Here's how the part is built. I have some questions about the finished solid (model axes, mm). A direction names the side the tool comes from. Give positions to 0.01 mm unless a question says otherwise; leave off trailing zeros. Order: outer loops, then holes, each group sorted by start corner. A loop starts at its lowest first (then second) coordinate and runs counter-clockwise, first axis right, second up.
from build123d import *

# Parameters (mm, degrees)
F0_R     = 25.4
F1_DEPTH = 142.875
F2_R     = 5.5626
F3_DEPTH = 6.35
F4_R     = 2.413
F5_DEPTH = 9.525


with BuildPart() as f1:
    # F0 (on Top) → F1 (new body)
    with BuildSketch(Plane.XY):
        Circle(F0_R)
    extrude(amount=F1_DEPTH)

    # F2 (on face) → F3 (join)
    with BuildSketch(Plane.XY.offset(142.875)):
        with Locations((-11.1125, 0)):
            Circle(F2_R)
    extrude(amount=F3_DEPTH)

    # F4 (on face) → F5 (cut)
    with BuildSketch(Plane.XY.offset(149.225)):
        with Locations((-11.1125, 0)):
            Circle(F4_R)
    extrude(amount=-F5_DEPTH, mode=Mode.SUBTRACT)

    # F6: F1 across plane


with BuildPart() as f1_1:
    add(f1.part)
    add(f1.part.mirror(Plane.YZ))


solid = f1_1.part
Q1. If we section it at D-D on x = 0: List the corners of the cut face in (y, z) for me (3 decimals), plus the area to 3 significant figures.
Filled sheet:
outline: (-25.4, 0) - (25.4, 0) - (25.4, 142.875) - (-25.4, 142.875) - close
area: 7,260 mm2
Q2. Thinking about a two-plate mould opening in X: for faces 3 (the face through (-5.807, 1.671, 146.006)), 4 (the face through (8.7, -1.2, 149.225)), 5 (the face through (-5.506, -24.796, 70.437)), which applies, released by +X, released by -X, zero draft, split by the parting line, or undercut?
Filled sheet:
face 3: undercut
face 4: zero draft
face 5: split by the parting line
Q3. If we section it at A-A on y = 0: List the corners of the cut face in (x, z) for me (1 decimal).
Filled sheet:
outline: (-25.4, 0) - (25.4, 0) - (25.4, 142.9) - (16.7, 142.9) - (16.7, 149.2) - (13.5, 149.2) - (13.5, 142.9) - (8.7, 142.9) - (8.7, 149.2) - (5.5, 149.2) - (5.5, 142.9) - (-5.5, 142.9) - (-5.5, 149.2) - (-8.7, 149.2) - (-8.7, 142.9) - (-13.5, 142.9) - (-13.5, 149.2) - (-16.7, 149.2) - (-16.7, 142.9) - (-25.4, 142.9) - close
Q4. If we section it at B-B on z = 83.5: List the corners of the cut face in (x, y) for me.
Filled sheet:
outline: circle Ø50.8 at (0, 0)
Q5. For faces 1 (the face through (0, 0, 0)), 2 (the face through (11, 0, 142.875)), which set-ups out of +Z, -Z, +X, -X, +Y, -Y let a thin tool reach every point of the face, with its end or its side?
Filled sheet:
face 1: -Z, +X, -X, +Y, -Y
face 2: +Z
Q6. I need wall thicknesses on L1, parallel to Z at x = 8.5, y = 12 (3 decimals); L2, parallel to Y at x = 21.5, z = 124.5; L3, parallel to Y at x = -6, z = 62. Which ranges of each line are inside material? Lowest first, please.
Filled sheet:
L1: z = 0 to 142.875
L2: y = -13.52 to 13.52
L3: y = -24.68 to 24.68
Q7. If we section it at C-C on x = -12: List the corners of the cut face in (y, z) for me (3 decimals).
Filled sheet:
outline: (-22.387, 0) - (22.387, 0) - (22.387, 142.875) - (5.491, 142.875) - (5.491, 149.225) - (2.244, 149.225) - (2.244, 142.875) - (-2.244, 142.875) - (-2.244, 149.225) - (-5.491, 149.225) - (-5.491, 142.875) - (-22.387, 142.875) - close
Q8. I'm going to push flat-ended pins straight in: P1, Ø4, axis at x = -14, z = 91, coming from the -Y side; P2, Ø6, axis at y = 4.5, z = 47.5, coming from the +X side; P3, Ø6, axis at x = -5, z = 45.5, coming from the +Y side. Where does each tip first touch, or does it pass through?
Filled sheet:
P1: stops at y = -22.39
P2: stops at x = 25.36
P3: stops at y = 25.32
